```python
from build123d import *

# Parameters (mm, degrees)
SKETCH1_W           = 50.8
SKETCH1_H           = 50.8
BOSS_EXTRUDE1_DEPTH = 5.08
FILLET1_R           = 10.16
SKETCH2_W           = 6.35
SKETCH2_H           = 16.51
CUT_EXTRUDE1_DEPTH  = 5.08


with BuildPart() as part:
    # Sketch1 → Boss-Extrude1 (new body)
    with BuildSketch(Plane(origin=(0, 0, 0), x_dir=(1, 0, 0), z_dir=(0, 1, 0))):
        Rectangle(SKETCH1_W, SKETCH1_H)
    extrude(amount=BOSS_EXTRUDE1_DEPTH)

    # Fillet1
    fillet1_edges = [part.edges().sort_by_distance(p)[0] for p in [
        (25.4, 2.54, 25.4),
        (-25.4, 2.54, 25.4),
        (-25.4, 2.54, -25.4),
        (25.4, 2.54, -25.4),
    ]]
    fillet(fillet1_edges, radius=FILLET1_R)

    # Sketch2 → Cut-Extrude1 (cut)
    with BuildSketch(Plane(origin=(0, 5.08, 0), x_dir=(1, 0, 0), z_dir=(0, 1, 0))):
        with Locations((22.225, 0)):
            Rectangle(SKETCH2_W, SKETCH2_H)
    cut_extrude1 = extrude(amount=-CUT_EXTRUDE1_DEPTH, mode=Mode.SUBTRACT)

    # Mirror1: Cut-Extrude1 across plane
    add(cut_extrude1.mirror(Plane(origin=(0, 0, 0), x_dir=(0, 0, 1), z_dir=(1, 0, 0))), mode=Mode.SUBTRACT)


solid = part.part
```
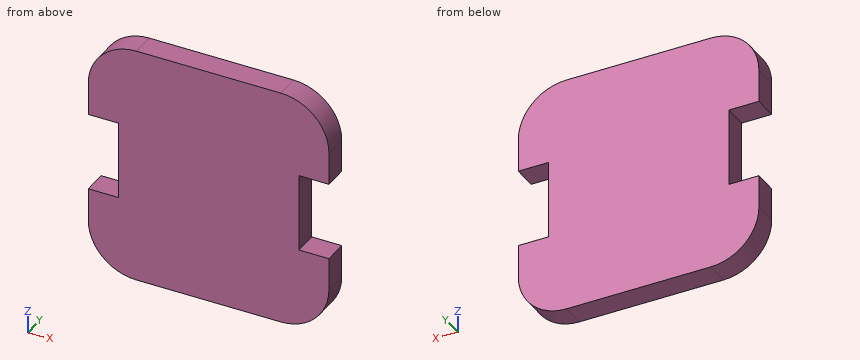
Here's how the part is built. I have some questions about the finished solid (model axes, mm). Round coordinates to 2 decimals unless told otherwise and drop trailing zeros. Order: outer loops, then holes, each group sorted by start corner. A loop starts at its lowest first (then second) coordinate and runs counter-clockwise, first axis right, second up. Notation, with made-up numbers: M 86.5,-36.75 L 94.5,-36.75 A13 cw 94.5,-13.75 Z; hole C 24.25,10.25 d5. An arc over 180 degrees is marked long. Answer in a Markdown table with one row per item.
Item 1: Imagine slicing it at A-A, the plane y = 1.15. Write out the boundary of the cut face in (x, z) (3 decimals).
A:
| item | result |
|---|---|
| outline | M -25.4,-15.24 A10.16 ccw -15.24,-25.4 L 15.24,-25.4 A10.16 ccw 25.4,-15.24 L 25.4,-8.255 L 19.05,-8.255 L 19.05,8.255 L 25.4,8.255 L 25.4,15.24 A10.16 ccw 15.24,25.4 L -15.24,25.4 A10.16 ccw -25.4,15.24 L -25.4,8.255 L -19.05,8.255 L -19.05,-8.255 L -25.4,-8.255 Z |
Item 2: If I drill on L1, parallel to X at y = 1.6, z = -5; L2, parallel to Z at x = 20, y = 1.3 (3 decimals); L3, parallel to Z at x = 20.5, y = 4.2 (3 decimals), over which ranges is the centre line in solid material (lowest first)? Write a range as from..to.
A:
| item | result |
|---|---|
| L1 | x = -19.05..19.05 |
| L2 | z = -24.216..-8.255, 8.255..24.216 |
| L3 | z = -23.932..-8.255, 8.255..23.932 |
Item 3: Imagine slicing it at C-C, the plane z = 6. Write out the boundary of the cut face in (x, y), and give its area (3 significant figures).
A:
| item | result |
|---|---|
| outline | M -19.05,0 L 19.05,0 L 19.05,5.08 L -19.05,5.08 Z |
| area | 194 mm2 |
Item 4: I'm going to push flat-ended pins straight in: pin 1 (1.5 mm diameter, centred on x = -22, y = 2, fed in from -Z); pin 2 (1.5 mm diameter, centred on x = 21.5, y = 3, fed in from +Z); pin 3 (1.5 mm diameter, centred on y = 3, z = 1, fed in from -X). Where does each tip first touch, or does it pass through?
A:
| item | result |
|---|---|
| pin 1 | stops at z = -23.43 |
| pin 2 | stops at z = 23.78 |
| pin 3 | stops at x = -19.05 |
Item 5: Imagine slicing it at B-B, the plane x = 20.5. Write out the boundary of the cut face in (y, z) (3 decimals).
A:
| item | result |
|---|---|
| outline | M 0,-23.932 L 5.08,-23.932 L 5.08,-8.255 L 0,-8.255 Z; M 0,8.255 L 5.08,8.255 L 5.08,23.932 L 0,23.932 Z |
